Check sheet for the modelled part. Datum: model origin and axes. Units: mm. A direction names the side the tool comes from. Round coordinates to 2 decimals unless told otherwise and drop trailing zeros. Loops run counter-clockwise (first coordinate to the right, second up) from the corner with the lowest first, then second, coordinate; pieces in that order, holes last. Notation, with made-up numbers: (76, -34.75) -> (116, -34.75) arc R22 ccw to (116, -11.75) -> close; hole circle Ø5 at (46.5, 27). An arc over 180 degrees is marked (long way). Return JSON: item names as keys, results as strings.
from build123d import *

# Parameters (mm, degrees)
F1_DEPTH = 25.4


with BuildPart() as f1:
    # F0 (on Top) → F1 (new body)
    with BuildSketch(Plane.XY):
        with BuildLine():
            ThreePointArc((49.313544, -12.198952), (50.427017, -6.144591), (50.8, 0))
            ThreePointArc((50.8, 0), (50.427017, 6.144591), (49.313544, 12.198952))
            ThreePointArc((49.313544, 12.198952), (49.069032, 13.148007), (48.806257, 14.09217))
            ThreePointArc((48.806257, 14.09217), (43.994091, 25.4), (36.607305, 35.221374))
            ThreePointArc((36.607305, 35.221374), (35.921024, 35.921024), (35.221374, 36.607305))
            ThreePointArc((35.221374, 36.607305), (25.4, 43.994091), (14.09217, 48.806257))
            ThreePointArc((14.09217, 48.806257), (13.148007, 49.069032), (12.198952, 49.313544))
            ThreePointArc((12.198952, 49.313544), (0, 50.8), (-12.198952, 49.313544))
            ThreePointArc((-12.198952, 49.313544), (-13.148007, 49.069032), (-14.09217, 48.806257))
            ThreePointArc((-14.09217, 48.806257), (-25.4, 43.994091), (-35.221374, 36.607305))
            ThreePointArc((-35.221374, 36.607305), (-35.921024, 35.921024), (-36.607305, 35.221374))
            ThreePointArc((-36.607305, 35.221374), (-43.994091, 25.4), (-48.806257, 14.09217))
            ThreePointArc((-48.806257, 14.09217), (-49.069032, 13.148007), (-49.313544, 12.198952))
            ThreePointArc((-49.313544, 12.198952), (-50.8, 0), (-49.313544, -12.198952))
            ThreePointArc((-49.313544, -12.198952), (-49.069032, -13.148007), (-48.806257, -14.09217))
            ThreePointArc((-48.806257, -14.09217), (-43.994091, -25.4), (-36.607305, -35.221374))
            ThreePointArc((-36.607305, -35.221374), (-35.921024, -35.921024), (-35.221374, -36.607305))
            ThreePointArc((-35.221374, -36.607305), (-25.4, -43.994091), (-14.09217, -48.806257))
            ThreePointArc((-14.09217, -48.806257), (-13.148007, -49.069032), (-12.198952, -49.313544))
            ThreePointArc((-12.198952, -49.313544), (0, -50.8), (12.198952, -49.313544))
            ThreePointArc((12.198952, -49.313544), (13.148007, -49.069032), (14.09217, -48.806257))
            ThreePointArc((14.09217, -48.806257), (25.4, -43.994091), (35.221374, -36.607305))
            ThreePointArc((35.221374, -36.607305), (35.921024, -35.921024), (36.607305, -35.221374))
            ThreePointArc((36.607305, -35.221374), (43.994091, -25.4), (48.806257, -14.09217))
            ThreePointArc((48.806257, -14.09217), (49.069032, -13.148007), (49.313544, -12.198952))
        make_face()
        with BuildLine():
            ThreePointArc((49.313544, 12.198952), (50.427017, 6.144591), (50.8, 0))
            ThreePointArc((50.8, 0), (50.427017, -6.144591), (49.313544, -12.198952))
            Line((49.313544, -12.198952), (73.66, 0))
            Line((73.66, 0), (49.313544, 12.198952))
        make_face()
        with BuildLine():
            ThreePointArc((36.607305, 35.221374), (43.994091, 25.4), (48.806257, 14.09217))
            Line((48.806257, 14.09217), (63.791431, 36.83))
            Line((63.791431, 36.83), (36.607305, 35.221374))
        make_face()
        with BuildLine():
            Line((63.791431, -36.83), (48.806257, -14.09217))
            ThreePointArc((48.806257, -14.09217), (43.994091, -25.4), (36.607305, -35.221374))
            Line((36.607305, -35.221374), (63.791431, -36.83))
        make_face()
        with BuildLine():
            ThreePointArc((14.09217, 48.806257), (25.4, 43.994091), (35.221374, 36.607305))
            Line((35.221374, 36.607305), (36.83, 63.791431))
            Line((36.83, 63.791431), (14.09217, 48.806257))
        make_face()
        with BuildLine():
            Line((36.83, -63.791431), (35.221374, -36.607305))
            ThreePointArc((35.221374, -36.607305), (25.4, -43.994091), (14.09217, -48.806257))
            Line((14.09217, -48.806257), (36.83, -63.791431))
        make_face()
        with BuildLine():
            ThreePointArc((-12.198952, 49.313544), (0, 50.8), (12.198952, 49.313544))
            Line((12.198952, 49.313544), (0, 73.66))
            Line((0, 73.66), (-12.198952, 49.313544))
        make_face()
        with BuildLine():
            Line((0, -73.66), (12.198952, -49.313544))
            ThreePointArc((12.198952, -49.313544), (0, -50.8), (-12.198952, -49.313544))
            Line((-12.198952, -49.313544), (0, -73.66))
        make_face()
        with BuildLine():
            ThreePointArc((-35.221374, 36.607305), (-25.4, 43.994091), (-14.09217, 48.806257))
            Line((-14.09217, 48.806257), (-36.83, 63.791431))
            Line((-36.83, 63.791431), (-35.221374, 36.607305))
        make_face()
        with BuildLine():
            Line((-36.83, -63.791431), (-14.09217, -48.806257))
            ThreePointArc((-14.09217, -48.806257), (-25.4, -43.994091), (-35.221374, -36.607305))
            Line((-35.221374, -36.607305), (-36.83, -63.791431))
        make_face()
        with BuildLine():
            ThreePointArc((-48.806257, 14.09217), (-43.994091, 25.4), (-36.607305, 35.221374))
            Line((-36.607305, 35.221374), (-63.791431, 36.83))
            Line((-63.791431, 36.83), (-48.806257, 14.09217))
        make_face()
        with BuildLine():
            Line((-63.791431, -36.83), (-36.607305, -35.221374))
            ThreePointArc((-36.607305, -35.221374), (-43.994091, -25.4), (-48.806257, -14.09217))
            Line((-48.806257, -14.09217), (-63.791431, -36.83))
        make_face()
        with BuildLine():
            ThreePointArc((-49.313544, -12.198952), (-50.8, 0), (-49.313544, 12.198952))
            Line((-49.313544, 12.198952), (-73.66, 0))
            Line((-73.66, 0), (-49.313544, -12.198952))
        make_face()
    extrude(amount=F1_DEPTH)


solid = f1.part
Q1. Section check B-B (x = -5). Record the boundary of the cut face in (y, z).
Results list:
{"outline": "(-63.68, 0) -> (63.68, 0) -> (63.68, 25.4) -> (-63.68, 25.4) -> close"}
Q2. Go/stop test with flat-tipped pins: pin 1 (4 mm diameter, centred on x = 54, z = 14, fed in from -Y); pin 2 (8 mm diameter, centred on x = 55, y = -12.5, fed in from +Z); pin 3 (1 mm diameter, centred on x = -5.5, z = 10.5, fed in from -Y); pin 4 (1.5 mm diameter, centred on y = -18.5, z = 14.5, fed in from +X). Record where each tip stops, or that it passes through.
Results list:
{"pin 1": "y = -36.37", "pin 2": "z = 25.4", "pin 3": "y = -63.68", "pin 4": "x = 52.21"}
Q3. Tool access check on faces 4 (the flat face through (6.014, -61.657, 12.522)), 5 (the flat face through (-61.657, -6.014, 12.522)), 6 (the flat face through (61.316, -6.185, 12.522)), 7 (the flat face through (-50.009, 36.014, 12.522)), 8 (the flat face through (-1, 1, 25.4)). Record the directions out of +Z, -Z, +X, -X, +Y, -Y that give a thin tool (end or side, any length) a straight path to the whole face; none if there is none.
Results list:
{"face 4": "+Z, -Z, -Y", "face 5": "+Z, -Z, -X", "face 6": "+Z, -Z, +X", "face 7": "+Z, -Z, +Y", "face 8": "+Z, +X, -X, +Y, -Y"}
Q4. Draft check along Y on faces 1 (the flat face through (36.037, -50.39, 12.522)), 2 (the flat face through (50.39, 36.037, 12.522)), 3 (the flat face through (-50.39, -36.037, 12.522)). Enter one of: released by +Y, released by -Y, zero draft, split by the parting line, or undercut.
Results list:
{"face 1": "undercut", "face 2": "released by +Y", "face 3": "released by -Y"}
Q5. Section check A-A (y = 53.5). Record the boundary of the cut face in (x, z), then the cut area to 3 significant figures.
Results list:
{"outline": "(-36.22, 0) -> (-21.21, 0) -> (-21.21, 25.4) -> (-36.22, 25.4) -> close; (-10.1, 0) -> (10.1, 0) -> (10.1, 25.4) -> (-10.1, 25.4) -> close; (21.21, 0) -> (36.22, 0) -> (36.22, 25.4) -> (21.21, 25.4) -> close", "area": "1,280 mm^2"}
Q6. Material ranges on line 1 (Y direction, x = -57, z = 13); line 2 (X direction, y = -55, z = 15.75); line 3 (Y direction, x = -60.5, z = 12), recorded low to high.
Results list:
{"line 1": "-36.43 to -26.52, -8.35 to 8.35, 26.52 to 36.43", "line 2": "-36.31 to -23.49, -9.35 to 9.35, 23.49 to 36.31", "line 3": "-36.64 to -31.84, -6.59 to 6.59, 31.84 to 36.64"}
Q7. Section check C-C (y = 29.5). Record the boundary of the cut face in (x, z), then the cut area to 3 significant figures.
Results list:
{"outline": "(-58.96, 0) -> (58.96, 0) -> (58.96, 25.4) -> (-58.96, 25.4) -> close", "area": "3,000 mm^2"}
